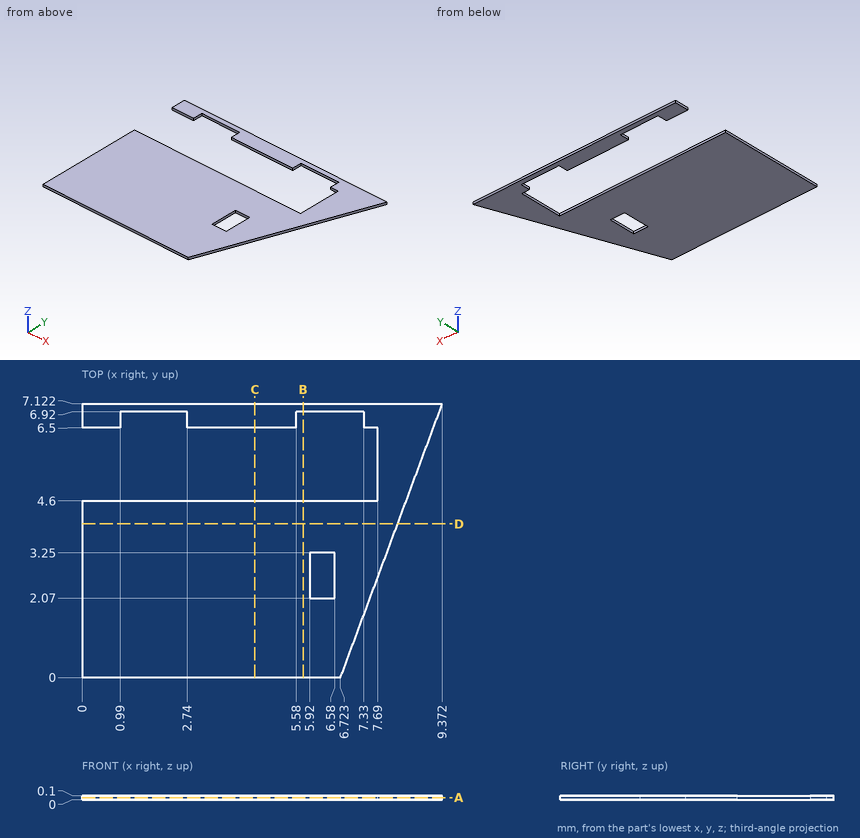
The figure shows three views and two pictorial views of one solid part (mm, origin at its lowest corner). Answer the questions. Coordinates: 2 decimals unless noted, no trailing zeros. Loops run counter-clockwise (first coordinate to the right, second up) from the corner with the lowest first, then second, coordinate; pieces in that order, holes last. Notation, with made-up numbers: (80.5, -38.75) -> (111.5, -38.75) arc R18 ccw to (111.5, -12.75) -> close; hole circle Ø8 at (2.5, -17). An arc over 180 degrees is marked (long way). Write item = value, one per line. Start each with the question number.
1) A cutting plane is placed at C-C (x = 4.5). Give the vertices of the cut face in (y, z).
2) A cutting plane is placed at A-A (z = 0.05). Give the vertices of the cut face in (x, y).
3) A cutting plane is placed at D-D (y = 4). Give the vertices of the cut face in (x, z).
4) Straight lines are drawn through the part: line 1 (Y direction, x = 6, z = 0.05); line 2 (Y direction, x = 2.5, z = 0.05); line 3 (Y direction, x = 5.5, z = 0.05). For each, find the intervals that lie inside material, in ascending order. Write a range as from..to.
5) A cutting plane is placed at B-B (x = 5.75). Give the vertices of the cut face in (y, z).
Responses:
q1.outline = (0, 0) -> (4.6, 0) -> (4.6, 0.1) -> (0, 0.1) -> close; (6.5, 0) -> (7.12, 0) -> (7.12, 0.1) -> (6.5, 0.1) -> close
q2.outline = (0, 0) -> (6.72, 0) -> (9.37, 7.12) -> (0, 7.12) -> (0, 6.5) -> (0.99, 6.5) -> (0.99, 6.92) -> (2.74, 6.92) -> (2.74, 6.5) -> (5.58, 6.5) -> (5.58, 6.92) -> (7.33, 6.92) -> (7.33, 6.5) -> (7.69, 6.5) -> (7.69, 4.6) -> (0, 4.6) -> close; hole (5.92, 2.07) -> (6.58, 2.07) -> (6.58, 3.25) -> (5.92, 3.25) -> close
q3.outline = (0, 0) -> (8.21, 0) -> (8.21, 0.1) -> (0, 0.1) -> close
q4.line_1 = 0..2.07, 3.25..4.6, 6.92..7.12
q4.line_2 = 0..4.6, 6.92..7.12
q4.line_3 = 0..4.6, 6.5..7.12
q5.outline = (0, 0) -> (4.6, 0) -> (4.6, 0.1) -> (0, 0.1) -> close; (6.92, 0) -> (7.12, 0) -> (7.12, 0.1) -> (6.92, 0.1) -> close
